```python
from build123d import *

# Parameters (mm, degrees)
BOSS_EXTRUDE1_DEPTH = 2.25
FILLET1_R           = 1


with BuildPart() as part:
    # Sketch1 → Boss-Extrude1 (new body, symmetric)
    with BuildSketch(Plane(origin=(0, 0, 0), x_dir=(1, 0, 0), z_dir=(0, 1, 0))):
        Polygon((-37.593296653, -44.5), (37.593296653, -44.5), (44.5, -27.233241632), (44.5, 27.233241632), (37.593296653, 44.5), (-37.593296653, 44.5), (-44.5, 27.233241632), (-44.5, -27.233241632), align=None)
        Polygon((-31.5, -35.5), (31.5, -35.5), (35.5, -25.5), (35.5, 25.5), (31.5, 35.5), (-31.5, 35.5), (-35.5, 25.5), (-35.5, -25.5), align=None, mode=Mode.SUBTRACT)
    extrude(amount=BOSS_EXTRUDE1_DEPTH, both=True)

    # Fillet1
    fillet1_edges = [part.edges().sort_by_distance(p)[0] for p in [
        (44.5, -2.25, 0),
        (41.046648326, -2.25, 35.866620816),
        (0, -2.25, 44.5),
        (-41.046648326, -2.25, 35.866620816),
        (41.046648326, 2.25, 35.866620816),
        (-44.5, 0, 27.233241632),
        (-44.5, 0, -27.233241632),
        (-37.593296653, 0, -44.5),
        (37.593296653, 0, -44.5),
        (44.5, 0, -27.233241632),
        (44.5, 0, 27.233241632),
        (37.593296653, 0, 44.5),
        (-37.593296653, 0, 44.5),
        (44.5, 2.25, 0),
        (41.046648326, 2.25, -35.866620816),
        (0, 2.25, -44.5),
        (33.5, -2.25, -30.5),
        (35.5, 0, -25.5),
        (0, -2.25, -35.5),
        (31.5, 0, -35.5),
        (-33.5, -2.25, -30.5),
        (-31.5, 0, -35.5),
        (-35.5, -2.25, 0),
        (-41.046648326, 2.25, -35.866620816),
        (-35.5, 0, -25.5),
        (-33.5, -2.25, 30.5),
        (-35.5, 0, 25.5),
        (0, -2.25, 35.5),
        (-31.5, 0, 35.5),
        (33.5, -2.25, 30.5),
        (31.5, 0, 35.5),
        (35.5, -2.25, 0),
        (35.5, 0, 25.5),
        (33.5, 2.25, -30.5),
        (0, 2.25, -35.5),
        (-33.5, 2.25, -30.5),
        (-35.5, 2.25, 0),
        (-33.5, 2.25, 30.5),
        (0, 2.25, 35.5),
        (33.5, 2.25, 30.5),
        (-44.5, 2.25, 0),
        (35.5, 2.25, 0),
        (-41.046648326, 2.25, 35.866620816),
        (-44.5, -2.25, 0),
        (0, 2.25, 44.5),
        (-41.046648326, -2.25, -35.866620816),
        (0, -2.25, -44.5),
        (41.046648326, -2.25, -35.866620816),
    ]]
    fillet(fillet1_edges, radius=FILLET1_R)


solid = part.part
```
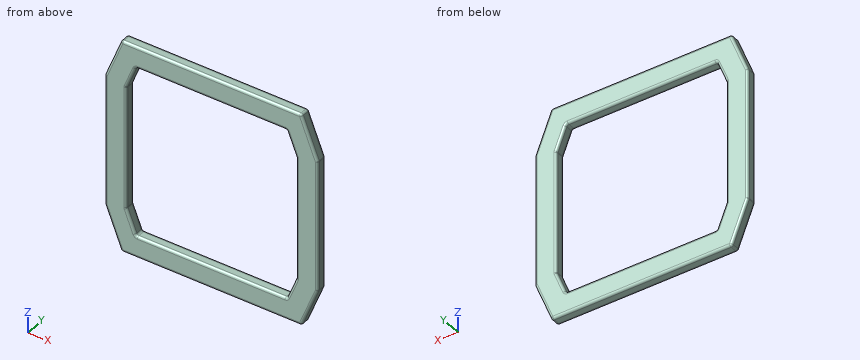
The model under review builds one solid part; all positions refer to its coordinate system, in mm. Round coordinates to 2 decimals unless told otherwise and drop trailing zeros. Loops run counter-clockwise (first coordinate to the right, second up) from the corner with the lowest first, then second, coordinate; pieces in that order, holes last.
Item 1: For line 1 (X direction, y = -0.2, z = 12.5); line 2 (Z direction, x = 31, y = 1.9), list the stretches that pass through material, from the lowest coordinate up.
Determined:
line 1: x = -44.5 to -35.5, 35.5 to 44.5
line 2: z = -44.26 to -35.73, 35.73 to 44.26
Item 2: Take a section at B-B (x = -3.5). Write out the cut boundary in (y, z).
Determined:
outline: (-2.25, -43.5) arc R1 ccw to (-1.25, -44.5) - (1.25, -44.5) arc R1 ccw to (2.25, -43.5) - (2.25, -36.5) arc R1 ccw to (1.25, -35.5) - (-1.25, -35.5) arc R1 ccw to (-2.25, -36.5) - close; (-2.25, 36.5) arc R1 ccw to (-1.25, 35.5) - (1.25, 35.5) arc R1 ccw to (2.25, 36.5) - (2.25, 43.5) arc R1 ccw to (1.25, 44.5) - (-1.25, 44.5) arc R1 ccw to (-2.25, 43.5) - close
Item 3: Take a section at A-A (z = -24). Write out the cut boundary in (x, y), then the cut area to 3 significant figures.
Determined:
outline: (-44.5, -1.25) arc R1 ccw to (-43.5, -2.25) - (-36.5, -2.25) arc R1 ccw to (-35.5, -1.25) - (-35.5, 1.25) arc R1 ccw to (-36.5, 2.25) - (-43.5, 2.25) arc R1 ccw to (-44.5, 1.25) - close; (35.5, -1.25) arc R1 ccw to (36.5, -2.25) - (43.5, -2.25) arc R1 ccw to (44.5, -1.25) - (44.5, 1.25) arc R1 ccw to (43.5, 2.25) - (36.5, 2.25) arc R1 ccw to (35.5, 1.25) - close
area: 79.3 mm2
Item 4: Clearance check with flat-ended pins moving along their axes: pin 1 Ø12 at (x, z) = (-7.5, -28) entering from -Y; pin 2 Ø12 at (x, z) = (-35.5, -17.5) entering from -Y. State where each tip first meets the part, or that it passes through.
Determined:
pin 1: passes through
pin 2: stops at y = -2.25
